Part model, mm, in its own coordinate system. A direction names the side the tool comes from. Coordinates: 2 decimals unless noted, no trailing zeros. Order: outer loops, then holes, each group sorted by start corner. A loop starts at its lowest first (then second) coordinate and runs counter-clockwise, first axis right, second up. Notation, with made-up numbers: (-31.5, 4) - (24.5, 4) arc R20 ccw to (24.5, 13) - close; hole circle Ø6 at (0.5, 3). An arc over 180 degrees is marked (long way). Use a Markdown table: item, result. Add a question column.
1) Two-plate mould, pull along X, no slides. Class faces 4 (the face through (28.976, 2.191, -0.861)), 5 (the face through (-30.467, 2.254, -4.997)), 6 (the face through (-0.3, 9.525, -0.1)): +X half, -X half, draft (parallel to the pull), parting line (faces both ways), or undercut.
2) Saw through at A-A on z = 0. List the corners of the cut face in (x, y) (3 decimals).
3) Tool access for faces 1 (the face through (-24, 4.445, 0)), 2 (the face through (24.6, 4.445, -1.3)), 3 (the face through (-29.146, 2.191, 0.099)): list every direction of +Z, -Z, +X, -X, +Y, -Y with a clear straight run to the whole face (end or side of a thin tool).
4) Saw through at D-D on x = -25.5. List the corners of the cut face in (y, z) (3 decimals), then the cut area to 3 significant figures.
5) Saw through at C-C on y = 6.75. List the corners of the cut face in (x, z), then the cut area to 3 significant figures.
6) Drop flat-ended pins along their axis: P1, Ø6, axis at x = 26.9, z = 0, coming from the +Y side (3 decimals); P2, Ø4, axis at y = 7, z = -2.5, coming from the +X side; P3, Ø5, axis at y = 8, z = 2.5, coming from the -X side. Give the stop position or say it passes through.
7) Wall check: L1, parallel to Z at x = 2.54, y = 7.25; L2, parallel to Z at x = 26.9, y = 3.5; L3, parallel to X at y = 0.75, z = 0.5. Give the ranges that are in metal, low to high. Write a range as [from, to].
8) Saw through at B-B on y = 3. List the corners of the cut face in (x, z), then the cut area to 3 significant figures.
```python
from build123d import *

# Parameters (mm, degrees)
SKETCH1_W               = 63.5
SKETCH1_H               = 12.7
EXTRUDE1_DEPTH          = 9.525
F_1_4_20_TAPPED_HOLE1_D = 5.1054
F_8_CLEARANCE_HOLE1_D   = 4.4958
SKETCH6_W               = 10
SKETCH6_H               = 12.7
CUT_EXTRUDE1_DEPTH      = 5.08
FILLET1_R               = 4.5


with BuildPart() as part:
    # Sketch1 → Extrude1 (new body)
    with BuildSketch(Plane(origin=(0, 0, 0), x_dir=(1, 0, 0), z_dir=(0, 1, 0))):
        Rectangle(SKETCH1_W, SKETCH1_H)
    extrude(amount=EXTRUDE1_DEPTH)

    # 1/4-20 Tapped Hole1 (through all)
    with Locations(Plane(origin=(-30.881531845, 9.525, 2.131635314), x_dir=(-1, 0, 0), z_dir=(0, 1, 0))):
        with Locations((-33.421531845, -2.131635314)):
            Hole(F_1_4_20_TAPPED_HOLE1_D / 2)

    # #8 Clearance Hole1 (through all)
    with Locations(Plane(origin=(34.21817196, 9.525, -1.204904774), x_dir=(-1, 0, 0), z_dir=(0, 1, 0))):
        with Locations((61.11817196, 1.204904774), (7.31817196, 1.204904774)):
            Hole(F_8_CLEARANCE_HOLE1_D / 2)

    # Sketch6 → Cut-Extrude1 (cut)
    with BuildSketch(Plane(origin=(0, 9.525, 0), x_dir=(-1, 0, 0), z_dir=(0, 1, 0))):
        with Locations((26.75, 0)):
            Rectangle(SKETCH6_W, SKETCH6_H)
        with Locations((-26.75, 0)):
            Rectangle(SKETCH6_W, SKETCH6_H)
    extrude(amount=-CUT_EXTRUDE1_DEPTH, mode=Mode.SUBTRACT)

    # Fillet1
    fillet1_edges = [part.edges().sort_by_distance(p)[0] for p in [
        (-31.75, 2.2225, -6.35),
        (-31.75, 2.2225, 6.35),
        (31.75, 2.2225, -6.35),
        (31.75, 2.2225, 6.35),
    ]]
    fillet(fillet1_edges, radius=FILLET1_R)


solid = part.part
```
Results are:
| question | item | result |
|---|---|---|
| 1 | face 4 | undercut |
| 1 | face 5 | -X half |
| 1 | face 6 | draft |
| 2 | outline | (-31.75, 0) - (-29.148, 0) - (-29.148, 4.445) - (-31.75, 4.445) - close; (-24.652, 0) - (-0.013, 0) - (-0.013, 9.525) - (-21.75, 9.525) - (-21.75, 4.445) - (-24.652, 4.445) - close; (5.093, 0) - (24.652, 0) - (24.652, 4.445) - (21.75, 4.445) - (21.75, 9.525) - (5.093, 9.525) - close; (29.148, 0) - (31.75, 0) - (31.75, 4.445) - (29.148, 4.445) - close |
| 3 | face 1 | +Z, -Z, -X, +Y |
| 3 | face 2 | +Z, -Z, +X, +Y |
| 3 | face 3 | +Y, -Y |
| 4 | outline | (0, -6.35) - (4.445, -6.35) - (4.445, -1.759) - (0, -1.759) - close; (0, 1.759) - (4.445, 1.759) - (4.445, 6.35) - (0, 6.35) - close |
| 4 | area | 40.8 mm2 |
| 5 | outline | (-21.75, -6.35) - (21.75, -6.35) - (21.75, 6.35) - (-21.75, 6.35) - close; hole circle Ø5.11 at (2.54, 0) |
| 5 | area | 532 mm2 |
| 6 | P1 | y = 4.445 |
| 6 | P2 | x = 21.75 |
| 6 | P3 | x = -21.75 |
| 7 | L1 | [-6.35, -2.55], [2.55, 6.35] |
| 7 | L2 | [-6.35, -2.25], [2.25, 6.35] |
| 7 | L3 | [-31.75, -29.09], [-24.71, 0.04], [5.04, 24.71], [29.09, 31.75] |
| 8 | outline | (-31.75, -1.85) arc R4.5 ccw to (-27.25, -6.35) - (27.25, -6.35) arc R4.5 ccw to (31.75, -1.85) - (31.75, 1.85) arc R4.5 ccw to (27.25, 6.35) - (-27.25, 6.35) arc R4.5 ccw to (-31.75, 1.85) - close; hole circle Ø4.5 at (-26.9, 0); hole circle Ø5.11 at (2.54, 0); hole circle Ø4.5 at (26.9, 0) |
| 8 | area | 737 mm2 |
